Verification items for the finished model (mm, model axes). A direction names the side the tool comes from. Coordinates: 2 decimals unless noted, no trailing zeros. Order: outer loops, then holes, each group sorted by start corner. A loop starts at its lowest first (then second) coordinate and runs counter-clockwise, first axis right, second up. Notation, with made-up numbers: (81.25, -35.75) - (118.25, -35.75) arc R30 cw to (118.25, -1.75) - close; hole circle Ø1 at (30.5, -26). An arc over 180 degrees is marked (long way). Answer as CSV lines item,"result". Start each with the question number.
1. Set-up check for faces 3 (the flat face through (30.33, 0, 56)), 4 (the flat face through (88.33, 0, -2)): record each of +Z, -Z, +X, -X, +Y, -Y from which the full face is reachable in a straight line by a thin tool's end or side.
2. Mould release check, pull along Z, two halves, no side actions. Record for faces 1 (the flat face through (-55, 0, -134.8)), 2 (the flat face through (-18, -3, 2)): pulls with the +Z half, pulls with the -Z half, needs draft (parallel to the pull), parting line crosses it, or undercut.
3. Material ranges on L1, parallel to X at y = 2.5, z = -61; L2, parallel to Z at x = 19.5, y = -1, recorded low to high. Write a range as [from, to].
4. Section check B-B (y = -0.8). Count the separate pieces of the cut face and the enclosed holes in it, and give its area (3 significant figures).
5. Section check A-A (z = 52.5). Record the cut outline in (x, y).
from build123d import *

# Parameters (mm, degrees)
F0_W     = 210
F0_H     = 297
F0_W_2   = 18
F0_H_2   = 43
F1_DEPTH = 3


with BuildPart() as f1:
    # F0 (on Front) → F1 (new body, symmetric)
    with BuildSketch(Plane.XZ):
        with Locations((-16.67, 0)):
            Rectangle(F0_W, F0_H)
        with Locations((-54.67, -113.3)):
            Rectangle(F0_W_2, F0_H_2, mode=Mode.SUBTRACT)
        with Locations((-54.67, -56.64)):
            Rectangle(F0_W_2, F0_H_2, mode=Mode.SUBTRACT)
        with Locations((21.33, -113.3)):
            Rectangle(F0_W_2, F0_H_2, mode=Mode.SUBTRACT)
        with Locations((21.33, -56.64)):
            Rectangle(F0_W_2, F0_H_2, mode=Mode.SUBTRACT)
        with Locations((-54.67, 0.02)):
            Rectangle(F0_W_2, F0_H_2, mode=Mode.SUBTRACT)
        with Locations((-54.67, 56.68)):
            Rectangle(F0_W_2, F0_H_2, mode=Mode.SUBTRACT)
        with Locations((-54.67, 113.34)):
            Rectangle(F0_W_2, F0_H_2, mode=Mode.SUBTRACT)
        with Locations((21.33, 0.02)):
            Rectangle(F0_W_2, F0_H_2, mode=Mode.SUBTRACT)
        with Locations((21.33, 56.68)):
            Rectangle(F0_W_2, F0_H_2, mode=Mode.SUBTRACT)
        with Locations((21.33, 113.34)):
            Rectangle(F0_W_2, F0_H_2, mode=Mode.SUBTRACT)
    extrude(amount=F1_DEPTH, both=True)


solid = f1.part
Evaluation:
1,face 3,"+Y, -Y"
1,face 4,"+Z, -Z, +X, +Y, -Y"
2,face 1,"undercut"
2,face 2,"needs draft"
3,L1,"x = [-121.67, -63.67], [-45.67, 12.33], [30.33, 88.33]"
3,L2,"z = [-148.5, -134.8], [-91.8, -78.14], [-35.14, -21.48], [21.52, 35.18], [78.18, 91.84], [134.84, 148.5]"
4,separate pieces,"1"
4,enclosed holes,"10"
4,area,"54,600 mm²"
5,outline,"(-121.67, -3) - (-63.67, -3) - (-63.67, 3) - (-121.67, 3) - close; (-45.67, -3) - (12.33, -3) - (12.33, 3) - (-45.67, 3) - close; (30.33, -3) - (88.33, -3) - (88.33, 3) - (30.33, 3) - close"
